CAD build for the part. Positions are in the model's coordinates, mm. Round coordinates to 2 decimals unless told otherwise and drop trailing zeros. Loops run counter-clockwise (first coordinate to the right, second up) from the corner with the lowest first, then second, coordinate; pieces in that order, holes last. Notation, with made-up numbers: M 79.25,55 L 137.25,55 A9 ccw 137.25,71 Z; hole C -0.75,22 d9. An arc over 180 degrees is marked long. Put each result on its own line as item: value. Start each with the question number.
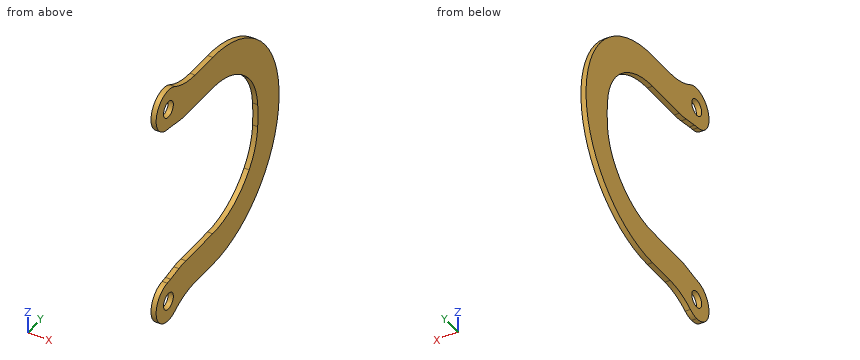
from build123d import *

# Parameters (mm, degrees)
BASE_FLANGE1_DEPTH          = 1.984375
F_1_4_0_25_DIAMETER_HOLE1_D = 6.35
BOSS_EXTRUDE1_DEPTH         = 1.984375
FILLET1_R                   = 25.4
CUT_EXTRUDE1_DEPTH          = 66.291667351
FILLET2_R                   = 25.4


# Sheet-metal steps are written as plain solids
with BuildPart() as part:
    # Sketch2 → Base-Flange1 (new body)
    with BuildSketch(Plane(origin=(0, 0, 0), x_dir=(0, 0, -1), z_dir=(1, 0, 0))):
        with BuildLine():
            Line((30.1625, 0), (30.1625, -28.575))
            ThreePointArc((30.1625, -28.575), (45.186761314, -36.352129933), (42.8625, -19.594743879))
            Line((42.8625, -19.594743879), (42.8625, 0))
            ThreePointArc((42.8625, 0), (0, 42.8625), (-42.8625, 0))
            Line((-42.8625, 0), (-42.8625, -19.594743879))
            ThreePointArc((-42.8625, -19.594743879), (-45.186761314, -36.352129933), (-30.1625, -28.575))
            Line((-30.1625, -28.575), (-30.1625, 0))
            ThreePointArc((-30.1625, 0), (0, 30.1625), (30.1625, 0))
        make_face()
    extrude(amount=-BASE_FLANGE1_DEPTH)

    # 1/4 (0.25) Diameter Hole1 (through all)
    with Locations(Plane(origin=(0, 0, 0), x_dir=(0, 0, -1), z_dir=(1, 0, 0))):
        with Locations((-39.6875, -28.575), (39.6875, -28.575)):
            Hole(F_1_4_0_25_DIAMETER_HOLE1_D / 2)

    # Sketch10 → Boss-Extrude1 (add)
    with BuildSketch(Plane(origin=(0, 0, 0), x_dir=(0, 0, -1), z_dir=(1, 0, 0))):
        with BuildLine():
            ThreePointArc((9.656385517, 28.575), (0, 30.1625), (-9.656385517, 28.575))
            ThreePointArc((-9.656385517, 28.575), (0, 29.207811784), (9.656385517, 28.575))
        make_face()
    extrude(amount=-BOSS_EXTRUDE1_DEPTH)

    # Fillet1
    fillet1_edges = [part.edges().sort_by_distance(p)[0] for p in [
        (-0.9921875, 28.575, 9.656385517),
        (-0.9921875, 28.575, -9.656385517),
    ]]
    fillet(fillet1_edges, radius=FILLET1_R)

    # Sketch11 → Cut-Extrude1 (cut, through all)
    with BuildSketch(Plane(origin=(0, 0, 0), x_dir=(0, 0, -1), z_dir=(1, 0, 0))):
        with BuildLine():
            Line((-42.8625, -21.300161084), (-42.8625, -19.594743879))
            ThreePointArc((-42.8625, -19.594743879), (-45.186761314, -36.352129933), (-30.1625, -28.575))
            Line((-30.1625, -28.575), (-30.1625, -19.594743879))
            Line((-30.1625, -19.594743879), (-31.75, -28.575))
            ThreePointArc((-31.75, -28.575), (-44.0350478, -35.215988961), (-42.8625, -21.300161084))
        make_face()
        with BuildLine():
            ThreePointArc((30.1625, -28.575), (45.186761314, -36.352129933), (42.8625, -19.594743879))
            Line((42.8625, -19.594743879), (42.8625, -21.300161084))
            ThreePointArc((42.8625, -21.300161084), (46.328488961, -24.2274522), (47.625, -28.575))
            ThreePointArc((47.625, -28.575), (39.6875, -36.5125), (31.75, -28.575))
            Line((31.75, -28.575), (30.1625, -19.594743879))
            Line((30.1625, -19.594743879), (30.1625, -28.575))
        make_face()
    extrude(amount=-CUT_EXTRUDE1_DEPTH, mode=Mode.SUBTRACT)

    # Fillet2
    fillet2_edges = [part.edges().sort_by_distance(p)[0] for p in [
        (-0.9921875, -21.300161084, 42.8625),
        (-0.9921875, -28.575, 31.75),
        (-0.9921875, -19.594743879, 30.1625),
        (-0.9921875, -28.575, -31.75),
        (-0.9921875, -21.300161084, -42.8625),
        (-0.9921875, -19.594743879, -30.1625),
    ]]
    fillet(fillet2_edges, radius=FILLET2_R)


solid = part.part
(1) Drill centre lines: line 1 along Z through (x, y) = (-1.4, -2.5); line 2 along Z through (x, y) = (-0.4, -20.5); line 3 along Z through (x, y) = (-0.85, -31.5). Where is each one in solid material? Low to high.
(2) Flat gauge pins, fed straight in: pin 1 Ø12 at (y, z) = (-11.5, -20) entering from +X; pin 2 Ø8.5 at (y, z) = (-28.58, -39.69) entering from +X; pin 3 Ø1 at (x, y) = (-1, -7.5) entering from -Z. Where does each tip first touch, or does it go through?
(3) Cut at B-B on y = -12.5. List the corners of the cut face in (x, z), and give its area (3 significant figures).
(4) Cut at D-D on z = 0. List the corners of the cut face in (x, y).
(5) Cut at C-C on x = -0.9. Count the separate pieces of the cut face and the enclosed holes in it, and give its area (3 significant figures).
(6) Cut at A-A on z = 40.5. List the corners of the cut face in (x, y).
Taken from the geometry:
1. line 1: -42.86 to -30.16, 30.16 to 42.86
1. line 2: -44.55 to -30.36, 30.36 to 44.55
1. line 3: -47.07 to -40.92, -38.45 to -32.31, 32.31 to 38.45, 40.92 to 47.07
2. pin 1: through
2. pin 2: x = 0
2. pin 3: z = -42.86
3. outline: M -1.98,-42.89 L 0,-42.89 L 0,-30.16 L -1.98,-30.16 Z; M -1.98,30.16 L 0,30.16 L 0,42.89 L -1.98,42.89 Z
3. area: 50.5 mm2
4. outline: M -1.98,29.21 L 0,29.21 L 0,42.86 L -1.98,42.86 Z
5. separate pieces: 1
5. enclosed holes: 2
5. area: 2,390 mm2
6. outline: M -1.98,-36.47 L 0,-36.47 L 0,-31.64 L -1.98,-31.64 Z; M -1.98,-25.51 L 0,-25.51 L 0,14.03 L -1.98,14.03 Z
